Here's how the part is built. I have some questions about the finished solid (model axes, mm). Face numbers are marked on the shaded views. A direction names the side the tool comes from. Give positions to 0.01 mm unless a question says otherwise; leave off trailing zeros. Write each loop counter-clockwise with the first axis right and the second up, starting at its lowest first coordinate (ties: lowest second). Pieces come first, ordered by that corner, then holes. Notation, with made-up numbers: (-36, 57.5) -> (-10, 57.5) arc R28 ccw to (-10, 92.5) -> close; hole circle Ø11 at (23, -1). An arc over 180 degrees is marked (long way). Return JSON: item names as keys, results as strings.
from build123d import *

# Parameters (mm, degrees)
BOSS_EXTRUDE1_DEPTH = 19
SKETCH2_W           = 33
SKETCH2_H           = 13
CUT_EXTRUDE1_DEPTH  = 3
CUT_EXTRUDE2_REACH  = 60.752
SKETCH3_W           = 23
SKETCH3_H           = 13
CUT_EXTRUDE3_REACH  = 60.752
SKETCH4_W           = 5
SKETCH4_H           = 5


with BuildPart() as part:
    # Sketch1 → Boss-Extrude1 (new body)
    with BuildSketch(Plane.XY):
        Polygon((-29.283593539, 0), (29.283593539, 0), (43.14, -24), (49.14, -24), (32.396842194, 5), (-32.396842194, 5), (-49.14, -24), (-43.14, -24), align=None)
    extrude(amount=BOSS_EXTRUDE1_DEPTH)

    # Sketch2 → Cut-Extrude1 (cut)
    with BuildSketch(Plane(origin=(0, 5, 0), x_dir=(1, 0, 0), z_dir=(0, 1, 0))):
        with Locations((-5.8, -9.5)):
            Rectangle(SKETCH2_W, SKETCH2_H)
    extrude(amount=-CUT_EXTRUDE1_DEPTH, mode=Mode.SUBTRACT)

    # Sketch3 → Cut-Extrude2 (cut, up to next)
    with BuildSketch(Plane(origin=(0, 2, 0), x_dir=(1, 0, 0), z_dir=(0, 1, 0)), mode=Mode.PRIVATE) as cut_extrude2_sk1:
        with Locations((-5.8, -9.5)):
            Rectangle(SKETCH3_W, SKETCH3_H)
    cut_extrude2_tool1 = extrude(cut_extrude2_sk1.sketch, amount=-CUT_EXTRUDE2_REACH, mode=Mode.PRIVATE) & part.part
    add(cut_extrude2_tool1.solids().sort_by_distance((-5.8, 2, 9.5))[0], mode=Mode.SUBTRACT)

    # Sketch4 → Cut-Extrude3 (cut, up to next)
    with BuildSketch(Plane(origin=(0, 2, 0), x_dir=(1, 0, 0), z_dir=(0, 1, 0)), mode=Mode.PRIVATE) as cut_extrude3_sk1:
        with Locations((8.2, -9.5)):
            Rectangle(SKETCH4_W, SKETCH4_H)
    cut_extrude3_tool1 = extrude(cut_extrude3_sk1.sketch, amount=-CUT_EXTRUDE3_REACH, mode=Mode.PRIVATE) & part.part
    add(cut_extrude3_tool1.solids().sort_by_distance((8.2, 2, 9.5))[0], mode=Mode.SUBTRACT)


solid = part.part
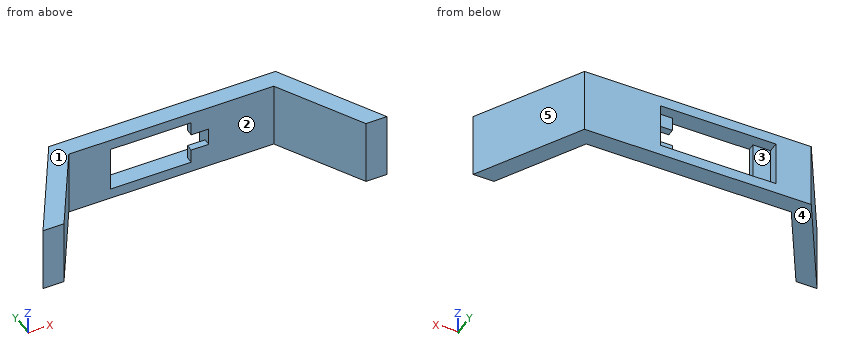
1. Suppose I cut it at A-A, the plane z = 13.25. List the corners of the cut face in (x, y) for me, and give its area (3 significant figures).
Taken from the geometry:
{"outline": "(-49.14, -24) -> (-43.14, -24) -> (-29.28, 0) -> (-17.3, 0) -> (-17.3, 2) -> (-22.3, 2) -> (-22.3, 5) -> (-32.4, 5) -> close; (5.7, 0) -> (29.28, 0) -> (43.14, -24) -> (49.14, -24) -> (32.4, 5) -> (10.7, 5) -> (10.7, 2) -> (5.7, 2) -> close", "area": "481 mm²"}
2. Which directions (+Z, -Z, +X, -X, +Y, -Y) give clear straight access to the entire face, cutting with the end or side of a thin tool? Please do the marked faces 1 and 2.
Taken from the geometry:
{"face 1": "+Z, +X, -X, +Y, -Y", "face 2": "+Z, -Z, -Y"}
3. Suppose I cut it at D-D, the plane z = 8.5. List the corners of the cut face in (x, y) for me, and give its area (3 significant figures).
Taken from the geometry:
{"outline": "(-49.14, -24) -> (-43.14, -24) -> (-29.28, 0) -> (-17.3, 0) -> (-17.3, 2) -> (-22.3, 2) -> (-22.3, 5) -> (-32.4, 5) -> close; (10.7, 0) -> (29.28, 0) -> (43.14, -24) -> (49.14, -24) -> (32.4, 5) -> (10.7, 5) -> close", "area": "471 mm²"}
4. If we mould it in two halves opening along X, with no side actions, what happens to the marked faces 3, 4 and 5? For each: released by +X, released by -X, zero draft, split by the parting line, or undercut.
Taken from the geometry:
{"face 3": "undercut", "face 4": "zero draft", "face 5": "released by +X"}
5. Suppose I cut it at B-B, the plane x = -12.5. List the corners of the cut face in (y, z) for me.
Taken from the geometry:
{"outline": "(0, 0) -> (5, 0) -> (5, 3) -> (0, 3) -> close; (0, 16) -> (5, 16) -> (5, 19) -> (0, 19) -> close"}
6. Suppose I cut it at C-C, the plane y = -13.5. List the corners of the cut face in (x, z) for me, and give its area (3 significant figures).
Taken from the geometry:
{"outline": "(-43.08, 0) -> (-37.08, 0) -> (-37.08, 19) -> (-43.08, 19) -> close; (37.08, 0) -> (43.08, 0) -> (43.08, 19) -> (37.08, 19) -> close", "area": "228 mm²"}
7. If I drill on line 1 (X direction, y = -10.5, z = 10); line 2 (X direction, y = -19, z = 12.5); line 3 (Y direction, x = -17.5, z = 1), over which ranges is the centre line in solid material (lowest first)? Write a range as [from, to].
Taken from the geometry:
{"line 1": "x = [-41.35, -35.35], [35.35, 41.35]", "line 2": "x = [-46.25, -40.25], [40.25, 46.25]", "line 3": "y = [0, 5]"}
8. For pin 1 Ø2 at (y, z) = (1.5, 13.5) entering from -X; pin 2 Ø1.6 at (y, z) = (1.5, 10) entering from +X; pin 3 Ø1.2 at (x, z) = (9, 15) entering from +Y, each with a flat end and sliding along its axis, tell me the tip position at first contact or that it passes through.
Taken from the geometry:
{"pin 1": "stops at x = -34.99", "pin 2": "stops at x = 34.88", "pin 3": "stops at y = 2"}
